Source: CAD feature listing. Evaluate the final solid. Frame: model axes, mm. A direction names the side the tool comes from. Round coordinates to 2 decimals unless told otherwise and drop trailing zeros. Loops run counter-clockwise (first coordinate to the right, second up) from the corner with the lowest first, then second, coordinate; pieces in that order, holes last. Notation, with made-up numbers: (57, -40) -> (107, -40) arc R24 ccw to (107, -9) -> close; hole circle Ø2 at (42, 55). An arc over 180 degrees is marked (long way). Return JSON: item names as keys, results as strings. Group by question number.
```python
from build123d import *

# Parameters (mm, degrees)
BOSS_EXTRUDE1_DEPTH = 2
FILLET1_R           = 0.5
BOSS_EXTRUDE2_DEPTH = 2
FILLET4_R           = 0.1
SKETCH3_R           = 1.5
BOSS_EXTRUDE3_DEPTH = 2
CUT_EXTRUDE4_DEPTH  = 2


with BuildPart() as part:
    # Sketch1 → Boss-Extrude1 (new body)
    with BuildSketch(Plane.XY):
        Polygon((-16, 16), (-16, 10), (-7, 10), (-7, 16), (10, 16), (10, 10), (17, 10), (17, 16), (22, 16), (22, -16), (-22, -16), (-22, 16), align=None)
    extrude(amount=BOSS_EXTRUDE1_DEPTH)

    # Fillet1
    fillet1_edges = [part.edges().sort_by_distance(p)[0] for p in [
        (22, 0, 0),
        (0, -16, 0),
        (-22, 0, 0),
        (-19, 16, 0),
        (-16, 13, 0),
        (-11.5, 10, 0),
        (-7, 13, 0),
        (1.5, 16, 0),
        (10, 13, 0),
        (13.5, 10, 0),
        (17, 13, 0),
        (19.5, 16, 0),
        (22, 16, 1),
        (1.5, 16, 2),
        (-22, 16, 1),
        (-16, 16, 1),
        (-7, 16, 1),
        (10, 16, 1),
        (17, 16, 1),
        (-19, 16, 2),
        (19.5, 16, 2),
    ]]
    fillet(fillet1_edges, radius=FILLET1_R)

    # Sketch2 → Boss-Extrude2 (add)
    with BuildSketch(Plane.XY.offset(2)):
        Polygon((20, 13.5), (19, 13.5), (19, 10.002928169), (8, 10.002928169), (8, 13.5), (-5, 13.5), (-5, 10), (-18, 10), (-18, 13.5), (-20, 13.5), (-20, -14), (20, -14), align=None)
        Polygon((7, 9.002928169), (19.458039892, 9.002928169), (19.458533352, -13), (19, -13), (-18.458039892, -13), (-18.458039892, 9.002928169), (-4, 9.002928169), (-4, 12.5), (7, 12.5), align=None, mode=Mode.SUBTRACT)
    extrude(amount=BOSS_EXTRUDE2_DEPTH)

    # Fillet4
    fillet4_edges = [part.edges().sort_by_distance(p)[0] for p in [
        (13.5, 10.002928169, 4),
        (8, 11.751464084, 4),
        (1.5, 13.5, 4),
        (-5, 11.75, 4),
        (-11.5, 10, 4),
        (-18, 11.75, 4),
        (-19, 13.5, 4),
        (-20, -0.25, 4),
        (0, -14, 4),
        (20, -0.25, 4),
        (19.5, 13.5, 4),
        (19, 11.751464084, 4),
        (-4, 10.751464084, 4),
        (-11.229019946, 9.002928169, 4),
        (-18.458039892, -1.998535916, 4),
        (0.50024673, -13, 4),
        (19.458286622, -1.998535916, 4),
        (13.229019946, 9.002928169, 4),
        (7, 10.751464084, 4),
        (1.5, 12.5, 4),
    ]]
    fillet(fillet4_edges, radius=FILLET4_R)

    # Sketch3 → Boss-Extrude3 (add)
    with BuildSketch(Plane.XY.offset(2)):
        with Locations((-11.329019946, 4)):
            Circle(SKETCH3_R)
        with Locations((-11.329019946, -4)):
            Circle(SKETCH3_R)
    extrude(amount=BOSS_EXTRUDE3_DEPTH)

    # Sketch4 → Cut-Extrude4 (cut)
    with BuildSketch(Plane.XY.offset(2)):
        with BuildLine():
            Line((16.189786245, 4.482679464), (15.482679464, 5.189786245))
            ThreePointArc((15.482679464, 5.189786245), (14.952349378, 5.189786245), (14.952349378, 4.65945616))
            Line((14.952349378, 4.65945616), (15.65945616, 3.952349378))
            ThreePointArc((15.65945616, 3.952349378), (16.189786245, 3.952349378), (16.189786245, 4.482679464))
        make_face()
        with BuildLine():
            Line((15.836232855, 1.300698949), (12.300698949, 4.836232855))
            ThreePointArc((12.300698949, 4.836232855), (11.770368863, 4.836232855), (11.770368863, 4.305902769))
            Line((11.770368863, 4.305902769), (15.305902769, 0.770368863))
            ThreePointArc((15.305902769, 0.770368863), (15.836232855, 0.770368863), (15.836232855, 1.300698949))
        make_face()
        with BuildLine():
            Line((16.01300955, -2.411611652), (8.588388348, 5.01300955))
            ThreePointArc((8.588388348, 5.01300955), (8.058058262, 5.01300955), (8.058058262, 4.482679464))
            Line((8.058058262, 4.482679464), (15.482679464, -2.941941738))
            ThreePointArc((15.482679464, -2.941941738), (16.01300955, -2.941941738), (16.01300955, -2.411611652))
        make_face()
        with BuildLine():
            Line((16.189786245, -6.123922254), (4.876077746, 5.189786245))
            ThreePointArc((4.876077746, 5.189786245), (4.345747661, 5.189786245), (4.345747661, 4.65945616))
            Line((4.345747661, 4.65945616), (15.65945616, -6.654252339))
            ThreePointArc((15.65945616, -6.654252339), (16.189786245, -6.654252339), (16.189786245, -6.123922254))
        make_face()
        with BuildLine():
            Line((0.633437059, 4.836232855), (15.836232855, -10.366562941))
            ThreePointArc((15.836232855, -10.366562941), (16.366562941, -10.366562941), (16.366562941, -9.836232855))
            Line((16.366562941, -9.836232855), (1.163767145, 5.366562941))
            ThreePointArc((1.163767145, 5.366562941), (0.633437059, 5.366562941), (0.633437059, 4.836232855))
        make_face()
        with BuildLine():
            ThreePointArc((0.810213755, 1.123922254), (0.810213755, 1.654252339), (1.34054384, 1.654252339))
            Line((1.34054384, 1.654252339), (12.654252339, -9.65945616))
            ThreePointArc((12.654252339, -9.65945616), (12.654252339, -10.189786245), (12.123922254, -10.189786245))
            Line((12.123922254, -10.189786245), (0.810213755, 1.123922254))
        make_face()
        with BuildLine():
            ThreePointArc((0.98699045, -2.588388348), (0.98699045, -2.058058262), (1.517320536, -2.058058262))
            Line((1.517320536, -2.058058262), (8.941941738, -9.482679464))
            ThreePointArc((8.941941738, -9.482679464), (8.941941738, -10.01300955), (8.411611652, -10.01300955))
            Line((8.411611652, -10.01300955), (0.98699045, -2.588388348))
        make_face()
        with BuildLine():
            ThreePointArc((1.163767145, -6.300698949), (1.163767145, -5.770368863), (1.694097231, -5.770368863))
            Line((1.694097231, -5.770368863), (5.229631137, -9.305902769))
            ThreePointArc((5.229631137, -9.305902769), (5.229631137, -9.836232855), (4.699301051, -9.836232855))
            Line((4.699301051, -9.836232855), (1.163767145, -6.300698949))
        make_face()
        with BuildLine():
            ThreePointArc((0.810213755, -9.482679464), (0.810213755, -8.952349378), (1.34054384, -8.952349378))
            Line((1.34054384, -8.952349378), (2.047650622, -9.65945616))
            ThreePointArc((2.047650622, -9.65945616), (2.047650622, -10.189786245), (1.517320536, -10.189786245))
            Line((1.517320536, -10.189786245), (0.810213755, -9.482679464))
        make_face()
    extrude(amount=-CUT_EXTRUDE4_DEPTH, mode=Mode.SUBTRACT)


solid = part.part
```
(1) Cut plane B-B (x = -5.5). Return loops of the section in (y, z).
(2) Set-up query: faces 5 (the face through (-18, 12, 3)), 6 (the face through (20, 0, 3)), 7 (the face through (6.546, -4.612, 1.014)). Return all of +Z, -Z, +X, -X, +Y, -Y with unobstructed straight access to the full face (end or side cutting, diameter ignored); none if empty.
(3) Pin query (flat end, axial travel): pin 1 (1 mm diameter, centred on x = 15, z = 3, fed in from +Y); pin 2 (0.5 mm diameter, centred on x = 19.5, z = 3.5, fed in from +Y); pin 3 (1 mm diameter, centred on x = 11, z = 3.5, fed in from -Y). Return the tip coordinate at first contact, or that it passes through.
(4) Ray query, line 1 (Y direction, x = 9.5, z = 2.65); line 2 (X direction, y = 10.5, z = 3.1); line 3 (X direction, y = -6, z = 2.45). Return the intervals inside material, ascending.
(5) Mould query, pull axis X, two halves, no side actions, for faces 1 (the face through (22, 0, 1)), 2 (the face through (1, 12.5, 3)), 3 (the face through (-19, 16, 1)), 4 (the face through (17, 13, 1)). Classes: released by +X, released by -X, zero draft, split by the parting line, or undercut.
(6) Cut plane C-C (y = -4). Count the separate pieces of the cut face and the enclosed holes in it, and give its area (3 significant figures).
(7) Cut plane A-A (z = 2.8). Return loops of the section in (x, y).
Answers follow:
{
 "1": {"outline": "(-16, 0.5) arc R0.5 ccw to (-15.5, 0) -> (15.5, 0) arc R0.5 ccw to (16, 0.5) -> (16, 1.5) arc R0.5 ccw to (15.5, 2) -> (10, 2) -> (10, 3.9) arc R0.1 ccw to (9.9, 4) -> (9.1, 4) arc R0.1 ccw to (9, 3.9) -> (9, 2) -> (-13, 2) -> (-13, 3.9) arc R0.1 ccw to (-13.1, 4) -> (-13.9, 4) arc R0.1 ccw to (-14, 3.9) -> (-14, 2) -> (-16, 2) -> close"},
 "2": {"face 5": "+Z, +Y", "face 6": "+Z, +X, +Y, -Y", "face 7": "+Z, -Z"},
 "3": {"pin 1": "y = 10", "pin 2": "y = 13.5", "pin 3": "y = -14"},
 "4": {"line 1": "-14 to -13, 9 to 10", "line 2": "-20 to -18, -5 to -4, 7 to 8, 19 to 20", "line 3": "-20 to -18.46, 19.46 to 20"},
 "5": {"face 1": "released by +X", "face 2": "undercut", "face 3": "zero draft", "face 4": "undercut"},
 "6": {"separate pieces": "5", "enclosed holes": "0", "area": "89.6 mm^2"},
 "7": {"outline": "(-20, -14) -> (20, -14) -> (20, 13.5) -> (19, 13.5) -> (19, 10) -> (8, 10) -> (8, 13.5) -> (-5, 13.5) -> (-5, 10) -> (-18, 10) -> (-18, 13.5) -> (-20, 13.5) -> close; circle Ø3 at (-11.33, -4); circle Ø3 at (-11.33, 4); hole (-18.46, -13) -> (19.46, -13) -> (19.46, 9) -> (7, 9) -> (7, 12.5) -> (-4, 12.5) -> (-4, 9) -> (-18.46, 9) -> close"}
}
